from build123d import *

# Parameters (mm, degrees)
SKETCH2_W           = 19.05
SKETCH2_H           = 76.2
SKETCH2_R           = 1.5875
BOSS_EXTRUDE1_DEPTH = 3.175
FILLET1_R           = 8.89
FILLET2_R           = 8.89


with BuildPart() as part:
    # Sketch2 → Boss-Extrude1 (new body)
    with BuildSketch(Plane(origin=(0, 0, 0), x_dir=(1, 0, 0), z_dir=(0, 1, 0))):
        Rectangle(SKETCH2_W, SKETCH2_H)
        with Locations((0, -25.4)):
            Circle(SKETCH2_R, mode=Mode.SUBTRACT)
    extrude(amount=BOSS_EXTRUDE1_DEPTH)

    # Fillet1
    fillet1_edges = [part.edges().sort_by_distance(p)[0] for p in [
        (9.525, 1.5875, 38.1),
    ]]
    fillet(fillet1_edges, radius=FILLET1_R)

    # Fillet2
    fillet2_edges = [part.edges().sort_by_distance(p)[0] for p in [
        (-9.525, 1.5875, 38.1),
    ]]
    fillet(fillet2_edges, radius=FILLET2_R)


solid = part.part
Geometry: final body of the model. Coordinates: model frame, mm. Coordinates: 2 decimals unless noted, no trailing zeros. Order: outer loops, then holes, each group sorted by start corner. A loop starts at its lowest first (then second) coordinate and runs counter-clockwise, first axis right, second up.
1) Section C-C (x = 0). Return loops of the section in (y, z) (1 decimal), then the cut area to 3 significant figures.
Result sheet:
outline: (0, -38.1) - (3.2, -38.1) - (3.2, 23.8) - (0, 23.8) - close; (0, 27) - (3.2, 27) - (3.2, 38.1) - (0, 38.1) - close
area: 232 mm2
2) Section D-D (x = -7.75). Return loops of the section in (y, z) (3 decimals).
Result sheet:
outline: (0, -38.1) - (3.175, -38.1) - (3.175, 34.54) - (0, 34.54) - close
3) Ray query, probe 1 along Z at (x, y) = (0, 2.15); probe 2 along X at (y, z) = (2.1, 25.4) (1 decimal); probe 3 along Z at (x, y) = (0.5, 0.7). Return the intervals inside material, ascending.
Result sheet:
probe 1: z = -38.1 to 23.81, 26.99 to 38.1
probe 2: x = -9.5 to -1.6, 1.6 to 9.5
probe 3: z = -38.1 to 23.89, 26.91 to 38.1
4) Section B-B (z = 25.4). Return loops of the section in (x, y) (1 decimal).
Result sheet:
outline: (-9.5, 0) - (-1.6, 0) - (-1.6, 3.2) - (-9.5, 3.2) - close; (1.6, 0) - (9.5, 0) - (9.5, 3.2) - (1.6, 3.2) - close
5) Section A-A (y = 2.5). Return loops of the section in (x, z) (1 decimal), then the cut area to 3 significant figures.
Result sheet:
outline: (-9.5, -38.1) - (9.5, -38.1) - (9.5, 29.2) arc R8.9 ccw to (0.6, 38.1) - (-0.6, 38.1) arc R8.9 ccw to (-9.5, 29.2) - close; hole circle Ø3.2 at (0, 25.4)
area: 1,410 mm2
6) Draft query along Z for faces 1 (the flat face through (9.525, 2, -4)), 2 (the cylindrical face through (0.85, 1.57, 24.06)), 3 (the flat face through (0, 2, -38.1)). Return one class per face: released by +Z, released by -Z, zero draft, split by the parting line, or undercut.
Result sheet:
face 1: zero draft
face 2: undercut
face 3: released by -Z
